For this review, take the finished solid that the model builds, in its own axes (mm). Round coordinates to 2 decimals unless told otherwise and drop trailing zeros. Order: outer loops, then holes, each group sorted by start corner. A loop starts at its lowest first (then second) coordinate and runs counter-clockwise, first axis right, second up.
Autodesk Inventor part; units mm, degrees
ref_plane "Work Plane1" through (0, 0, 7) normal (0, 0, 1) x (1, 0, 0)
ref_plane "Work Plane2" through (0, 0, 11) normal (0, 0, 1) x (1, 0, 0)
ref_plane "Work Plane3" through (0, 0, -20.5) normal (0, 0, 1) x (1, 0, 0)
sketch "Sketch1" plane through (0, 0, 0) normal (0, 0, 1) x (1, 0, 0)
  line L0 (15.9491, 0) -> (16.0494, 0)
  line L1 (-19.8, 0) -> (19.8, 0)
  arc A0 (19.8, 0) -> (-19.8, 0) centre (0, 0) ccw
  dimension "d32" = 39.6
ref_plane "Work Plane1" through (0, 0, 7) normal (0, 0, 1) x (1, 0, 0)
revolve "Revolution3" add sketch "Sketch1" angle 360 about axis through (15.9491, 0, 0) along (1, 0, 0)
ref_plane "Work Plane2" through (0, 0, 11) normal (0, 0, 1) x (1, 0, 0)
sketch "Sketch17" plane through (0, 0, 0) normal (0, 1, 0) x (-1, 0, 0)
  line L0 (26.807, 7) -> (13.1257, 7)
  line L1 (13.1257, 7) -> (3.4348, 21.8215)
  line L2 (3.4348, 21.8215) -> (26.807, 7)
  point P0 (0, 0)
  dimension "d50" = 7
extrude "Extrusion10" cut sketch "Sketch17" along normal through all both and the other way through all
shell "Shell4" thickness 0.5 removed faces 2 at (-15.7431, -1.7688, 7) at (-10.8801, -4.3558, 10.4345)
sketch "Sketch16" plane through (0, 0, 0) normal (0, 1, 0) x (-1, 0, 0)
  circle A0 centre (0, 0) radius 1.55
  dimension "d39" = 3.1
extrude "Extrusion9" cut sketch "Sketch16" along normal through all both and the other way through all
sketch "Sketch18" plane through (0, 0, 0) normal (1, 0, 0) x (0, 1, 0)
  circle A0 centre (0, 0) radius 1
  dimension "d46" = 2
extrude "Extrusion11" cut sketch "Sketch18" against normal through all
ref_plane "Work Plane3" through (0, 0, -20.5) normal (0, 0, 1) x (1, 0, 0)
properties part number "ping pong ball"
(1) Draft analysis for pull direction Y (two halves, no side actions). For faces 1 (the face through (-18.2, -0.1, 7)), 2 (the face through (-19.521, -0.217, -0.976)), state which applies: pulls with the +Y half, pulls with the -Y half, needs draft (parallel to the pull), parting line crosses it, or undercut.
(2) Clearance check with flat-ended pins moving along their axes: P1, Ø8, axis at x = -3.5, y = -10.5, coming from the +Z side; P2, Ø4, axis at y = -7, z = 5, coming from the +X side; P3, Ø5, axis at y = -11.5, z = 11, coming from the -X side. State where each tip first meets the part, or that it passes through.
(3) Add section A-A on z = 0. Give the boundary of the cut face in (x, y), plus the area to 3 significant figures.
(4) Add section D-D on z = -15.5. Give the boundary of the cut face in (x, y).
(5) Wall thickness on L1, parallel to Y at x = -0.5, z = 9; L2, parallel to Y at x = -3.5, z = -9.5; L3, parallel to X at y = 3, z = -1: over which ranges is each line inside the solid? List them lowest first.
(6) Add section C-C on y = 0. Give the boundary of the cut face in (x, z).
(7) Add section B-B on x = 0. Give the boundary of the cut face in (y, z), plus the area to 3 significant figures.
Here are the results:
1. face 1: needs draft
1. face 2: undercut
2. P1: stops at z = 18.5
2. P2: stops at x = 18.67
2. P3: stops at x = -12.05
3. outline: (-19.77, -1) arc R19.8 ccw to (-1.55, -19.74) - (-1.55, -19.24) arc R19.3 cw to (-19.27, -1) - close; (-19.77, 1) - (-19.27, 1) arc R19.3 cw to (-1.55, 19.24) - (-1.55, 19.74) arc R19.8 ccw to start; (1.55, -19.74) arc R19.8 ccw to (1.55, 19.74) - (1.55, 19.24) arc R19.3 cw to (1.55, -19.24) - close
3. area: 57.3 mm2
4. outline: circle Ø24.64 at (0, 0); hole circle Ø23 at (0, 0)
5. L1: y = -17.63 to -17.07, 17.07 to 17.63
5. L2: y = -17.02 to -16.43, 16.43 to 17.02
5. L3: x = -19.55 to -19.04, 19.04 to 19.55
6. outline: (-19.77, -1) arc R19.8 ccw (long way) to (-5.21, 19.1) - (-5.63, 18.46) arc R19.3 cw (long way) to (-19.27, -1) - close; (-19.77, 1) - (-19.27, 1) arc R19.3 cw to (-17.99, 7) - (-18.52, 7) arc R19.8 ccw to start
7. outline: (-19.74, -1.55) arc R19.8 ccw to (19.74, -1.55) - (19.24, -1.55) arc R19.3 cw to (-19.24, -1.55) - close; (-19.74, 1.55) - (-19.24, 1.55) arc R19.3 cw to (19.24, 1.55) - (19.74, 1.55) arc R19.8 ccw to start
7. area: 58.3 mm2
